CAD build for the part. Positions are in the model's coordinates, mm. A direction names the side the tool comes from. Round coordinates to 2 decimals unless told otherwise and drop trailing zeros. Order: outer loops, then holes, each group sorted by start corner. A loop starts at its lowest first (then second) coordinate and runs counter-clockwise, first axis right, second up. Notation, with made-up numbers: M -38.5,79.5 L -13.5,79.5 A20 ccw -13.5,98.5 Z; hole C -2,7 d5. An arc over 180 degrees is marked long. Put each result on its own line as item: value.
```python
from build123d import *

# Parameters (mm, degrees)
SKETCH1_R           = 4.95
BOSS_EXTRUDE1_DEPTH = 6
SKETCH2_R           = 5.5
BOSS_EXTRUDE2_DEPTH = 4
SKETCH3_R           = 15
BOSS_EXTRUDE3_DEPTH = 14.5
SKETCH4_R           = 4.3
BOSS_EXTRUDE4_DEPTH = 1.5
BOSS_EXTRUDE5_DEPTH = 4.5
SKETCH6_R           = 1.5
BOSS_EXTRUDE6_DEPTH = 17.5


with BuildPart() as part:
    # Sketch1 → Boss-Extrude1 (new body)
    with BuildSketch(Plane(origin=(0, 0, 0), x_dir=(1, 0, 0), z_dir=(0, 1, 0))):
        with Locations(Location((0, 0, 0), (0, 0, 270))):
            Circle(SKETCH1_R)
    extrude(amount=BOSS_EXTRUDE1_DEPTH)

    # Sketch2 → Boss-Extrude2 (add)
    with BuildSketch(Plane(origin=(0, 6, 0), x_dir=(1, 0, 0), z_dir=(0, 1, 0))):
        with Locations(Location((0, 0, 0), (0, 0, 270))):
            Circle(SKETCH2_R)
    extrude(amount=BOSS_EXTRUDE2_DEPTH)

    # Sketch3 → Boss-Extrude3 (add)
    with BuildSketch(Plane(origin=(0, 10, 0), x_dir=(1, 0, 0), z_dir=(0, 1, 0))):
        with Locations(Location((0, 0, 0), (0, 0, 90))):
            Circle(SKETCH3_R)
    extrude(amount=BOSS_EXTRUDE3_DEPTH)

    # Sketch4 → Boss-Extrude4 (add)
    with BuildSketch(Plane(origin=(0, 24.5, 0), x_dir=(1, 0, 0), z_dir=(0, 1, 0))):
        with Locations(Location((0, 0, 0), (0, 0, 270))):
            Circle(SKETCH4_R)
    extrude(amount=BOSS_EXTRUDE4_DEPTH)

    # Sketch5 → Boss-Extrude5 (add)
    with BuildSketch(Plane(origin=(0, 26, 0), x_dir=(1, 0, 0), z_dir=(0, 1, 0))):
        with BuildLine():
            Line((-3.3, 2.75680975), (-3.3, -2.75680975))
            ThreePointArc((-3.3, -2.75680975), (0, -4.3), (3.3, -2.75680975))
            Line((3.3, -2.75680975), (3.3, 2.75680975))
            ThreePointArc((3.3, 2.75680975), (0, 4.3), (-3.3, 2.75680975))
        make_face()
    extrude(amount=BOSS_EXTRUDE5_DEPTH)

    # Sketch6 → Boss-Extrude6 (add)
    with BuildSketch(Plane(origin=(0, 30.5, 0), x_dir=(1, 0, 0), z_dir=(0, 1, 0))):
        with Locations(Location((0, 0, 0), (0, 0, 270))):
            Circle(SKETCH6_R)
    extrude(amount=BOSS_EXTRUDE6_DEPTH)


solid = part.part
```
Item 1: Band-saw the part on B-B on x = 0. Give the cut face in (y, z), and give its area (4 significant figures).
Answers below:
outline: M 0,-4.95 L 6,-4.95 L 6,-5.5 L 10,-5.5 L 10,-15 L 24.5,-15 L 24.5,-4.3 L 30.5,-4.3 L 30.5,-1.5 L 48,-1.5 L 48,1.5 L 30.5,1.5 L 30.5,4.3 L 24.5,4.3 L 24.5,15 L 10,15 L 10,5.5 L 6,5.5 L 6,4.95 L 0,4.95 Z
area: 642.5 mm²
Item 2: Band-saw the part on C-C on y = 21. Give the cut face in (x, z).
Answers below:
outline: C 0,0 d30
Item 3: Band-saw the part on A-A on z = 0. Give the cut face in (x, y), and give its area (4 significant figures).
Answers below:
outline: M -15,10 L -5.5,10 L -5.5,6 L -4.95,6 L -4.95,0 L 4.95,0 L 4.95,6 L 5.5,6 L 5.5,10 L 15,10 L 15,24.5 L 4.3,24.5 L 4.3,26 L 3.3,26 L 3.3,30.5 L 1.5,30.5 L 1.5,48 L -1.5,48 L -1.5,30.5 L -3.3,30.5 L -3.3,26 L -4.3,26 L -4.3,24.5 L -15,24.5 Z
area: 633.5 mm²
Item 4: Probe line 1 along Y through (x, z) = (-12.75, -6.5); line 2 along X through (y, z) = (29.5, -2.5); line 3 along X through (y, z) = (31, 0). List the from-to ranges inside material, lowest first. Write a range as [from, to].
Answers below:
line 1: [10, 24.5]
line 2: [-3.3, 3.3]
line 3: [-1.5, 1.5]
Item 5: Tool access for faces 1 (the flat face through (3.3, 28, 0)), 2 (the flat face through (-4, 26, 0)), 3 (the cylindrical face through (-5.37, 7.97, -1.19)), 4 (the flat face through (0, 48, 0)), 5 (the flat face through (-4, 24.5, -3)): list every direction of +Z, -Z, +X, -X, +Y, -Y with a clear straight run to the whole face (end or side of a thin tool).
Answers below:
face 1: +Z, -Z, +X, +Y
face 2: +Z, -Z, -X, +Y
face 3: -Y
face 4: +Z, -Z, +X, -X, +Y
face 5: +Y
Item 6: Mould opens along Y. For faces 6 (the flat face through (-3.3, 28, 0)), 7 (the flat face through (4, 26, 0)), 8 (the flat face through (0, 0, 0)) say: pulls with the +Y half, pulls with the -Y half, needs draft (parallel to the pull), parting line crosses it, or undercut.
Answers below:
face 6: needs draft
face 7: pulls with the +Y half
face 8: pulls with the -Y half
Item 7: Band-saw the part on D-D on y = 40.5. Give the cut face in (x, z).
Answers below:
outline: C 0,0 d3
Item 8: Pin check, flat tips, straight feed: P1, Ø5, axis at x = -10.5, y = 11.5, coming from the -Z side; P2, Ø1, axis at y = 20, z = -2, coming from the +X side; P3, Ø3, axis at x = 6.5, z = -4.5, coming from the +Y side. Stop position of each tip, or through.
Answers below:
P1: z = -12.69
P2: x = 14.92
P3: y = 24.5
